The listing builds one solid part. Answer for the finished solid, in the listing's coordinates (mm). A direction names the side the tool comes from. Coordinates: 2 decimals unless noted, no trailing zeros. Order: outer loops, then holes, each group sorted by start corner. A loop starts at its lowest first (then second) coordinate and runs counter-clockwise, first axis right, second up. Notation, with made-up numbers: (-7.75, 82) -> (17.25, 82) arc R21 cw to (17.25, 109) -> close; hole circle Ø3 at (52.25, -14.5). An arc over 180 degrees is marked (long way). Put each result on its own line as item: value. Start each with the question number.
```python
from build123d import *

# Parameters (mm, degrees)
F1_DEPTH = 63.5
F0_W     = 28.432126
F0_H     = 12.001499
F2_DEPTH = 7.9375
F0_W_2   = 18.334983
F0_H_2   = 4.7498
F3_DEPTH = 25.4
F5_R     = 6.35


with BuildPart() as f1:
    # F0 (on Front) → F1 (new body, symmetric)
    with BuildSketch(Plane.XZ):
        Polygon((-41.275, 9.525), (-41.275, -9.525), (41.275, -9.525), (41.275, 9.525), (22.225, 9.525), align=None)
    extrude(amount=F1_DEPTH, both=True)

    # F0 (on Front) → F2 (join, symmetric)
    with BuildSketch(Plane.XZ):
        with BuildLine():
            add(Edge.make_bspline(
                [(-41.275, 9.525), (-27.868627, 39.151042), (-7.652168, 57.55358), (52.874146, 61.662466)],
                knots=[0, 0, 0, 0, 108.977586, 108.977586, 108.977586, 108.977586], degree=3))
            Line((-41.275, 9.525), (22.225, 9.525))
            Line((22.225, 9.525), (22.225, 27.0002))
            ThreePointArc((22.225, 27.0002), (30.986191, 50.134821), (52.874146, 61.662466))
        make_face()
        with Locations((-0.836268, 21.359812)):
            Rectangle(F0_W, F0_H, mode=Mode.SUBTRACT)
    extrude(amount=F2_DEPTH, both=True)

    # F0 (on Front) → F3 (join, symmetric)
    with BuildSketch(Plane.XZ):
        with BuildLine():
            Line((22.225, 9.525), (41.275, 9.525))
            Line((41.275, 9.525), (41.275, 27.0002))
            ThreePointArc((41.275, 27.0002), (45.92468, 38.22552), (57.15, 42.8752))
            Line((57.15, 42.8752), (67.390017, 42.8752))
            Line((67.390017, 42.8752), (67.390017, 61.9252))
            Line((67.390017, 61.9252), (57.15, 61.9252))
            add(Edge.make_bspline(
                [(52.874146, 61.662466), (54.277618, 61.757742), (55.702763, 61.845333), (57.15, 61.9252)],
                knots=[108.977586, 108.977586, 108.977586, 108.977586, 111.504536, 111.504536, 111.504536, 111.504536], degree=3))
            ThreePointArc((52.874146, 61.662466), (30.986191, 50.134821), (22.225, 27.0002))
            Line((22.225, 27.0002), (22.225, 9.525))
        make_face()
        with Locations((76.557508, 64.3001)):
            Rectangle(F0_W_2, F0_H_2)
    extrude(amount=F3_DEPTH, both=True)

    # F0 (on Front) → F4 (revolve)
    with BuildSketch(Plane.XZ):
        Polygon((85.725, 66.675), (85.725, 61.9252), (85.725, 42.8752), (85.725, 38.1), (118.190017, 38.1), (118.190017, 66.675), align=None)
    revolve(axis=Axis((85.725, 0, 52.4002), (0, 0, 1)))

    # F5
    f5_edges = [f1.edges().sort_by_distance(p)[0] for p in [
        (-41.275, -63.5, 0),
        (41.275, -63.5, 0),
        (41.275, 63.5, 0),
        (-41.275, 63.5, 0),
    ]]
    fillet(f5_edges, radius=F5_R)


solid = f1.part
```
(1) The part is cut by section C-C on x = 79. Determine the outline of the cut face in (y, z) (3 decimals).
(2) The part is cut by section A-A on z = 3. Determine the outline of the cut face in (x, y) (3 decimals), plus the area to 3 significant figures.
(3) Each of these flat-tipped pins is pushed along its axis until it touches: P1, Ø5, axis at x = -6, z = 25, coming from the -Y side; P2, Ø2, axis at y = 6, z = 56.5, coming from the +X side; P3, Ø12, axis at x = 77.5, y = -7, coming from the -Z side. Where does it stop, or does it pass through?
(4) The part is cut by section B-B on y = -35.5. Determine the outline of the cut face in (x, z) (3 decimals), plus the area to 3 significant figures.
(5) A tool of negligible diameter and unlimited length cuts with its end or side. For faces 1 (the cylindrical face through (31.222, 16.547, 50.399)), 2 (the flat face through (86, 0, 38.1)), 3 (the flat face through (59, -23, 42.875)), 4 (the flat face through (-4, -7.938, 30)), from which of +Z, -Z, +X, -X, +Y, -Y can it reach the whole face along a straight path? Write none if from no direction.
(6) Find the intervals of material crossed by L1, parallel to Z at x = 5, y = 48.5 (3 decimals); L2, parallel to X at y = 23.5, z = 11 (3 decimals); L3, parallel to X at y = 18, z = -5.5 (3 decimals), in increasing order.
(7) For a pull along X with two mould halves and no side action, classify faces 5 (the flat face through (13.38, 0, 21)), 6 (the flat face through (-41.275, -1, 0)), 7 (the cylindrical face through (39.464, -61.59, 0.133)) as released by +X, released by -X, zero draft, split by the parting line, or undercut.
Worked out:
1. outline: (-31.761, 38.1) -> (31.761, 38.1) -> (31.761, 66.675) -> (-31.761, 66.675) -> close
2. outline: (-41.275, -57.15) arc R6.35 ccw to (-34.925, -63.5) -> (34.925, -63.5) arc R6.35 ccw to (41.275, -57.15) -> (41.275, 57.15) arc R6.35 ccw to (34.925, 63.5) -> (-34.925, 63.5) arc R6.35 ccw to (-41.275, 57.15) -> close
2. area: 10,400 mm2
3. P1: y = -7.94
3. P2: x = 117.8
3. P3: z = 38.1
4. outline: (-41.275, -9.525) -> (41.275, -9.525) -> (41.275, 9.525) -> (-41.275, 9.525) -> close
4. area: 1,570 mm2
5. face 1: +Z, -X, +Y
5. face 2: -Z, +X, +Y, -Y
5. face 3: -Z, -Y
5. face 4: +Z, -X, -Y
6. L1: -9.525 to 9.525
6. L2: 22.225 to 41.275
6. L3: -41.275 to 41.275
7. face 5: undercut
7. face 6: released by -X
7. face 7: released by +X
